```python
from build123d import *

# Parameters (mm, degrees)
SKETCH_1_W               = 25
SKETCH_1_H               = 50
SKETCH_1_R               = 1.5
EXTRUDE_1_DEPTH          = 3
EXTRUDE_START            = 22
EXTRUDE_2_DEPTH          = 3
CUT_EXTRUDE_1_DEPTH      = 3
CUT_EXTRUDE_2_DEPTH      = 3
RIB_1_REACH              = 70.903
SKETCH_7_WALL_W          = 152.805886826
SKETCH_7_WALL_H          = 3
PATTERN_CIRCULAR_1_COUNT = 2
SKETCH_8_W               = 25
SKETCH_8_H               = 3
EXTRUDE_3_DEPTH          = 50
SKETCH_9_W               = 12
SKETCH_9_H               = 5
EXTRUDE_4_DEPTH          = 50
SKETCH_10_W              = 3
SKETCH_10_H              = 45
EXTRUDE_5_DEPTH          = 3


with BuildPart() as part:
    # Sketch 1 → Extrude 1 (new body)
    with BuildSketch(Plane.XY):
        Rectangle(SKETCH_1_W, SKETCH_1_H)
        with Locations((0, 18.5)):
            Circle(SKETCH_1_R, mode=Mode.SUBTRACT)
        with Locations(Location((0, -18.5, 0), (0, 0, 180))):
            Circle(SKETCH_1_R, mode=Mode.SUBTRACT)
    extrude(amount=EXTRUDE_1_DEPTH)

    # Sketch 4 → Extrude 2 (add)
    with BuildSketch(Plane(origin=(0, 0, 0), x_dir=(1, 0, 0), z_dir=(0, 1, 0)).offset(EXTRUDE_START)):
        with BuildLine():
            Line((-22.5, -3), (22.5, -3))
            Line((22.5, -3), (37.725646944, 32.188161826))
            ThreePointArc((37.725646944, 32.188161826), (0, 40), (-37.725646944, 32.188161826))
            Line((-37.725646944, 32.188161826), (-22.5, -3))
        make_face()
    extrude_2 = extrude(amount=EXTRUDE_2_DEPTH)

    # Mirror 1: Extrude 2 across plane
    add(extrude_2.mirror(Plane.ZX))

    # Sketch 5 → Cut-Extrude 1 (cut)
    with BuildSketch(Plane.XZ.offset(25)):
        Polygon((0, 0), (12.5, 0), (12.5, 3), (39.027541645, 3), (39.027541645, -43.548502894), (0, -43.548502894), align=None)
    extrude(amount=-CUT_EXTRUDE_1_DEPTH, mode=Mode.SUBTRACT)

    # Sketch 6 → Cut-Extrude 2 (cut)
    with BuildSketch(Plane(origin=(0, 25, 0), x_dir=(1, 0, 0), z_dir=(0, 1, 0))):
        Polygon((0, 0), (-12.5, 0), (-12.5, -3), (-39.063803434, -3), (-39.063803434, 42.915846613), (0, 42.915846613), align=None)
    extrude(amount=-CUT_EXTRUDE_2_DEPTH, mode=Mode.SUBTRACT)

    # Sketch 7 wall → Rib 1 (add, up to next)
    with BuildSketch(Plane(origin=(-12.5, -16, -2.5), x_dir=(0, 0.923076923077, 0.384615384615), z_dir=(0, 0.384615384615, -0.923076923077)), mode=Mode.PRIVATE) as rib_1_sk1:
        with Locations((0, 1.5)):
            Rectangle(SKETCH_7_WALL_W, SKETCH_7_WALL_H)
    rib_1_tool1 = extrude(rib_1_sk1.sketch, amount=-RIB_1_REACH, mode=Mode.PRIVATE) - part.part
    rib_1 = rib_1_tool1.solids().sort_by_distance((-12.5, -16, -2.5))[0]
    add(rib_1)

    # Pattern Circular 1: Rib 1 ×2 about axis
    pattern_circular_1_axis = Axis((0, 0, -26.4), (0, 0, 1))
    for i in range(1, PATTERN_CIRCULAR_1_COUNT):
        add(rib_1.rotate(pattern_circular_1_axis, i * 360 / PATTERN_CIRCULAR_1_COUNT))

    # Sketch 8 → Extrude 3 (add)
    with BuildSketch(Plane(origin=(0, 25, 0), x_dir=(1, 0, 0), z_dir=(0, 1, 0))):
        with Locations((0, -1.5)):
            Rectangle(SKETCH_8_W, SKETCH_8_H)
    extrude(amount=EXTRUDE_3_DEPTH)

    # Sketch 9 → Extrude 4 (add)
    with BuildSketch(Plane(origin=(0, 0, 0), x_dir=(-1, 0, 0), z_dir=(0, 0, -1))):
        with Locations((0, 72.5)):
            Rectangle(SKETCH_9_W, SKETCH_9_H)
    extrude(amount=EXTRUDE_4_DEPTH)

    # Sketch 10 → Extrude 5 (add)
    with BuildSketch(Plane(origin=(0, 0, 0), x_dir=(-1, 0, 0), z_dir=(0, 0, -1))):
        with Locations((-4.5, 47.5)):
            Rectangle(SKETCH_10_W, SKETCH_10_H)
        with Locations((4.5, 47.5)):
            Rectangle(SKETCH_10_W, SKETCH_10_H)
    extrude(amount=EXTRUDE_5_DEPTH)


solid = part.part
```
CAD build for the part. Positions are in the model's coordinates, mm. A direction names the side the tool comes from. Give positions to 0.01 mm unless a question says otherwise; leave off trailing zeros. Loops run counter-clockwise (first coordinate to the right, second up) from the corner with the lowest first, then second, coordinate; pieces in that order, holes last. Notation, with made-up numbers: (68, -2.5) - (86, -2.5) arc R12 ccw to (86, 8.5) - close; hole circle Ø7 at (45, 25). An arc over 180 degrees is marked (long way). Put each result on its own line as item: value.
Q1. Flat gauge pins, fed straight in: pin 1 (2.5 mm diameter, centred on y = 62, z = 1, fed in from +X); pin 2 (12 mm diameter, centred on y = 35, z = -12, fed in from -X); pin 3 (5 mm diameter, centred on x = 7.5, y = 57.5, fed in from -Z); pin 4 (1.5 mm diameter, centred on y = 16, z = -2.5, fed in from -X). Where does each tip first touch, or does it go through?
Filled in:
pin 1: stops at x = 12.5
pin 2: passes through
pin 3: stops at z = -3
pin 4: stops at x = 9.5
Q2. Mould opens along X. For faces 4 (the face through (-12.5, 15, 2)), 5 (the face through (-3, 13, 0)), 6 (the face through (19.53, 23.48, -37.97)) say: pulls with the +X half, pulls with the -X half, needs draft (parallel to the pull), parting line crosses it, or undercut.
Filled in:
face 4: pulls with the -X half
face 5: undercut
face 6: pulls with the +X half
Q3. Slice it at C-C (y = 60.5). Give the cut face in (x, z), plus the area to 3 significant figures.
Filled in:
outline: (-12.5, 0) - (-6, 0) - (-6, -3) - (-3, -3) - (-3, 0) - (3, 0) - (3, -3) - (6, -3) - (6, 0) - (12.5, 0) - (12.5, 3) - (-12.5, 3) - close
area: 93.0 mm²
Q4. Slice it at B-B (z = -9.5). Give the cut face in (x, y), plus the area to 3 significant figures.
Filled in:
outline: (-27.91, -25) - (0, -25) - (0, -22) - (-27.91, -22) - close; (-6, 70) - (6, 70) - (6, 75) - (-6, 75) - close; (0, 22) - (27.91, 22) - (27.91, 25) - (0, 25) - close
area: 227 mm²
Q5. Slice it at A-A (y = 18.5). Give the cut face in (x, z).
Filled in:
outline: (-12.5, 0) - (-1.5, 0) - (-1.5, 3) - (-12.5, 3) - close; (1.5, 0) - (9.5, 0) - (9.5, -3.54) - (12.5, -3.54) - (12.5, 3) - (1.5, 3) - close
Q6. Probe line 1 along Y through (x, z) = (0, 1.5); line 2 along X through (y, z) = (-18.5, 1.8); line 3 along Y through (x, z) = (5, -15.5). List the from-to ranges inside material, lowest first.
Filled in:
line 1: y = -25 to -20, -17 to 17, 20 to 75
line 2: x = -12.5 to -1.5, 1.5 to 12.5
line 3: y = 22 to 25, 70 to 75
Q7. Tool access for faces 1 (the face through (-4, 25, -1)), 2 (the face through (12.5, 50, 2)), 3 (the face through (3, 47, -1)): list every direction of +Z, -Z, +X, -X, +Y, -Y with a clear straight run to the whole face (end or side of a thin tool).
Filled in:
face 1: -Z, -X
face 2: +Z, -Z, +X, +Y
face 3: -Z
Q8. Slice it at D-D (x = 26.5). Give the cut face in (y, z).
Filled in:
outline: (22, -36.23) - (25, -36.23) - (25, -6.24) - (22, -6.24) - close
